from build123d import *

# Parameters (mm, degrees)
SKETCH1_R                = 3.95
BOSS_EXTRUDE1_DEPTH      = 49.15
M5_CLEARANCE_HOLE1_D     = 5.5
M5_CLEARANCE_HOLE1_DEPTH = 49.15
M5_CLEARANCE_HOLE1_TIP   = 1.652366702
FILLET1_R                = 0.2


with BuildPart() as part:
    # Sketch1 → Boss-Extrude1 (new body)
    with BuildSketch(Plane(origin=(0, 0, 0), x_dir=(1, 0, 0), z_dir=(0, 1, 0))):
        with Locations(Location((0, 0, 0), (0, 0, 270))):
            Circle(SKETCH1_R)
    extrude(amount=BOSS_EXTRUDE1_DEPTH)

    # M5 Clearance Hole1
    with Locations(Plane(origin=(0, 49.15, 0), x_dir=(1, 0, 0), z_dir=(0, 1, 0))):
        with Locations((0, 0)):
            Hole(M5_CLEARANCE_HOLE1_D / 2, depth=M5_CLEARANCE_HOLE1_DEPTH)
            with Locations((0, 0, -(M5_CLEARANCE_HOLE1_DEPTH + M5_CLEARANCE_HOLE1_TIP / 2))):  # 118° drill point
                Cone(0, M5_CLEARANCE_HOLE1_D / 2, M5_CLEARANCE_HOLE1_TIP, mode=Mode.SUBTRACT)

    # Fillet1
    fillet1_edges = [part.edges().sort_by_distance(p)[0] for p in [
        (0, 0, -3.95),
        (0, 49.15, -3.95),
        (2.75, 49.15, 0),
        (2.75, 0, 0),
    ]]
    fillet(fillet1_edges, radius=FILLET1_R)


solid = part.part
The model under review builds one solid part; all positions refer to its coordinate system, in mm. Give positions to 0.01 mm unless a question says otherwise; leave off trailing zeros. Write each loop counter-clockwise with the first axis right and the second up, starting at its lowest first coordinate (ties: lowest second). Pieces come first, ordered by that corner, then holes. Notation, with made-up numbers: M 22,32.25 L 43,32.25 A38 cw 43,71.25 Z; hole C 80.25,7 d11. An arc over 180 degrees is marked long. One line per question, with ' | ' between items. Start each with the question number.
Item 1: We need section A-A on x = 0. Write out the cut boundary in (y, z), plus the area to 3 significant figures.
Item 2: We need section C-C on y = 32.5. Write out the cut boundary in (x, z), plus the area to 3 significant figures.
Item 3: Draft analysis for pull direction X (two halves, no side actions). For faces 1 (the cylindrical face through (2.67, 24.23, -2.91)), 2 (the cylindrical face through (0.596, 24.234, 2.685)), 3 (the flat face through (-1, 0, -3)), state which applies: released by +X, released by -X, zero draft, split by the parting line, or undercut.
Item 4: We need section B-B on z = 0. Write out the cut boundary in (x, y).
Item 5: Wall thickness on line 1 (X direction, y = 34, z = 0); line 2 (Z direction, x = 2, y = 19); line 3 (Z direction, x = 1.75, y = 42): over which ranges is each line inside the solid? List them lowest first. Write a range as from..to.
Item 6: For pin 1 (2 mm diameter, centred on x = -2, y = 35, fed in from +Z); pin 2 (1.5 mm diameter, centred on x = 2, z = -1, fed in from -Y), all flat-tipped, find the tip position at first contact; note any pin that passes through.
Results found:
1) outline: M 0,-3.75 A0.2 ccw 0.2,-3.95 L 48.95,-3.95 A0.2 ccw 49.15,-3.75 L 49.15,-2.95 A0.2 ccw 48.95,-2.75 L 0.2,-2.75 A0.2 ccw 0,-2.95 Z; M 0,2.95 A0.2 ccw 0.2,2.75 L 48.95,2.75 A0.2 ccw 49.15,2.95 L 49.15,3.75 A0.2 ccw 48.95,3.95 L 0.2,3.95 A0.2 ccw 0,3.75 Z | area: 118 mm2
2) outline: C 0,0 d7.9; hole C 0,0 d5.5 | area: 25.3 mm2
3) face 1: split by the parting line | face 2: undercut | face 3: zero draft
4) outline: M -3.95,0.2 A0.2 ccw -3.75,0 L -2.95,0 A0.2 ccw -2.75,0.2 L -2.75,48.95 A0.2 ccw -2.95,49.15 L -3.75,49.15 A0.2 ccw -3.95,48.95 Z; M 2.75,0.2 A0.2 ccw 2.95,0 L 3.75,0 A0.2 ccw 3.95,0.2 L 3.95,48.95 A0.2 ccw 3.75,49.15 L 2.95,49.15 A0.2 ccw 2.75,48.95 Z
5) line 1: x = -3.95..-2.75, 2.75..3.95 | line 2: z = -3.41..-1.89, 1.89..3.41 | line 3: z = -3.54..-2.12, 2.12..3.54
6) pin 1: stops at z = 3.82 | pin 2: stops at y = 0
